from build123d import *

# Parameters (mm, degrees)
SKETCH2_W           = 127
SKETCH2_H           = 88.9
SKETCH2_R           = 6.35
SKETCH2_R_2         = 2.667
BOSS_EXTRUDE1_DEPTH = 12.7
FILLET1_R           = 6.35


with BuildPart() as part:
    # Sketch2 → Boss-Extrude1 (new body)
    with BuildSketch(Plane(origin=(0, 0, 0), x_dir=(1, 0, 0), z_dir=(0, 1, 0))):
        with Locations((0, -5.297057788)):
            Rectangle(SKETCH2_W, SKETCH2_H)
        with Locations(Location((-44.45, 13.752942212, 0), (0, 0, 270))):
            Circle(SKETCH2_R, mode=Mode.SUBTRACT)
        with Locations(Location((0, 26.452942212, 0), (0, 0, 270))):
            Circle(SKETCH2_R_2, mode=Mode.SUBTRACT)
        with Locations(Location((0, 13.752942212, 0), (0, 0, 270))):
            Circle(SKETCH2_R_2, mode=Mode.SUBTRACT)
        with Locations(Location((44.45, 13.752942212, 0), (0, 0, 270))):
            Circle(SKETCH2_R, mode=Mode.SUBTRACT)
        with Locations(Location((0, -37.047057788, 0), (0, 0, 270))):
            Circle(SKETCH2_R_2, mode=Mode.SUBTRACT)
        with Locations(Location((0, -24.347057788, 0), (0, 0, 270))):
            Circle(SKETCH2_R_2, mode=Mode.SUBTRACT)
    extrude(amount=BOSS_EXTRUDE1_DEPTH)

    # Fillet1
    fillet1_edges = [part.edges().sort_by_distance(p)[0] for p in [
        (-63.5, 6.35, 49.747057788),
        (-63.5, 6.35, -39.152942212),
        (63.5, 6.35, -39.152942212),
        (63.5, 6.35, 49.747057788),
    ]]
    fillet(fillet1_edges, radius=FILLET1_R)


solid = part.part
Source: CAD feature listing. Evaluate the final solid. Frame: model axes, mm. Coordinates: 2 decimals unless noted, no trailing zeros. Loops run counter-clockwise (first coordinate to the right, second up) from the corner with the lowest first, then second, coordinate; pieces in that order, holes last. Notation, with made-up numbers: (-5.75, 9) - (47.25, 9) arc R26 cw to (47.25, 43) - close; hole circle Ø7 at (34.25, 69). An arc over 180 degrees is marked (long way). One line per item, written item: value. Start each with the question number.
1. Section C-C (y = 7.25). Return the cut outline in (x, z), and give its area (3 significant figures).
2. Ray query, L1, parallel to Z at x = 2, y = 9; L2, parallel to Z at x = -43.5, y = 11.5; L3, parallel to X at y = 3.75, z = 25. Return the intervals inside material, ascending.
3. Section A-A (x = 0). Return the cut outline in (y, z).
4. Section B-B (x = 44.45). Return the cut outline in (y, z), and give its area (3 significant figures).
5. Mould query, pull axis X, two halves, no side actions, for faces 1 (the flat face through (-1, 6, -39.153)), 2 (the cylindrical face through (-1.62, 6.26, 34.93)), 3 (the cylindrical face through (61.59, 6.439, 47.936)). Classes: pulls with the +X half, pulls with the -X half, needs draft (parallel to the pull), parting line crosses it, or undercut.
Verdict:
1. outline: (-63.5, -32.8) arc R6.35 ccw to (-57.15, -39.15) - (57.15, -39.15) arc R6.35 ccw to (63.5, -32.8) - (63.5, 43.4) arc R6.35 ccw to (57.15, 49.75) - (-57.15, 49.75) arc R6.35 ccw to (-63.5, 43.4) - close; hole circle Ø12.7 at (-44.45, -13.75); hole circle Ø5.33 at (0, -26.45); hole circle Ø5.33 at (0, -13.75); hole circle Ø5.33 at (0, 24.35); hole circle Ø5.33 at (0, 37.05); hole circle Ø12.7 at (44.45, -13.75)
1. area: 10,900 mm2
2. L1: z = -39.15 to -28.22, -24.69 to -15.52, -11.99 to 22.58, 26.11 to 35.28, 38.81 to 49.75
2. L2: z = -39.15 to -20.03, -7.47 to 49.75
2. L3: x = -63.5 to -2.59, 2.59 to 63.5
3. outline: (0, -39.15) - (12.7, -39.15) - (12.7, -29.12) - (0, -29.12) - close; (0, -23.79) - (12.7, -23.79) - (12.7, -16.42) - (0, -16.42) - close; (0, -11.09) - (12.7, -11.09) - (12.7, 21.68) - (0, 21.68) - close; (0, 27.01) - (12.7, 27.01) - (12.7, 34.38) - (0, 34.38) - close; (0, 39.71) - (12.7, 39.71) - (12.7, 49.75) - (0, 49.75) - close
4. outline: (0, -39.15) - (12.7, -39.15) - (12.7, -20.1) - (0, -20.1) - close; (0, -7.4) - (12.7, -7.4) - (12.7, 49.75) - (0, 49.75) - close
4. area: 968 mm2
5. face 1: needs draft
5. face 2: undercut
5. face 3: pulls with the +X half
